from build123d import *

# Parameters (mm, degrees)
F0_R          = 3
F1_DEPTH      = 61
F1_DEPTH_BACK = 4
F0_R_2        = 5
F2_DEPTH      = 55
F5_D          = 2.5
F5_DEPTH      = 8
F5_TIP        = 0.7510757738
F6_D          = 3.5
F6_DEPTH      = 8
F6_TIP        = 1.0515060833


with BuildPart() as f1:
    # F0 (on Top) → F1 (new body, two sides)
    with BuildSketch(Plane.XY) as f1_sk:
        Circle(F0_R)
    extrude(amount=F1_DEPTH)
    extrude(f1_sk.sketch, amount=-F1_DEPTH_BACK)

    # F0 (on Top) → F2 (join)
    with BuildSketch(Plane.XY):
        Circle(F0_R_2)
        Circle(F0_R, mode=Mode.SUBTRACT)
    extrude(amount=F2_DEPTH)

    # F5
    with Locations(Plane(origin=(0, 0, -4), x_dir=(1, 0, 0), z_dir=(0, 0, -1))):
        with Locations((0, 0)):
            Hole(F5_D / 2, depth=F5_DEPTH)
            with Locations((0, 0, -(F5_DEPTH + F5_TIP / 2))):  # 118° drill point
                Cone(0, F5_D / 2, F5_TIP, mode=Mode.SUBTRACT)

    # F6
    with Locations(Plane.XY.offset(61)):
        with Locations((0, 0)):
            Hole(F6_D / 2, depth=F6_DEPTH)
            with Locations((0, 0, -(F6_DEPTH + F6_TIP / 2))):  # 118° drill point
                Cone(0, F6_D / 2, F6_TIP, mode=Mode.SUBTRACT)


solid = f1.part
Part model, mm, in its own coordinate system. A direction names the side the tool comes from. Round coordinates to 2 decimals unless told otherwise and drop trailing zeros. Order: outer loops, then holes, each group sorted by start corner. A loop starts at its lowest first (then second) coordinate and runs counter-clockwise, first axis right, second up. Notation, with made-up numbers: (18.5, 74.5) -> (32.5, 74.5) arc R26 ccw to (32.5, 93.5) -> close; hole circle Ø4 at (-18, -21). An arc over 180 degrees is marked (long way). Put each result on its own line as item: value.
Q1. Pull direction X, two halves, no side cores. Call faces 4 (the face through (-1.617, -0.67, 56.944)), 5 (the face through (-3, 0, 58)), 6 (the face through (-0.1, -3.3, 0)): pulls with the +X half, pulls with the -X half, needs draft (parallel to the pull), parting line crosses it, or undercut.
From the geometry:
face 4: undercut
face 5: parting line crosses it
face 6: needs draft
Q2. Band-saw the part on A-A (z = 26.5). Give the cut face in (x, y).
From the geometry:
outline: circle Ø10 at (0, 0)
Q3. Band-saw the part on B-B (x = 4.25). Give the cut face in (y, z).
From the geometry:
outline: (-2.63, 0) -> (2.63, 0) -> (2.63, 55) -> (-2.63, 55) -> close
Q4. Tool access for faces 1 (the face through (1, -1, -4)), 2 (the face through (0.27, 1.22, 0.06)), 3 (the face through (-0.1, -3.3, 55)): list every direction of +Z, -Z, +X, -X, +Y, -Y with a clear straight run to the whole face (end or side of a thin tool).
From the geometry:
face 1: -Z, +X, -X, +Y, -Y
face 2: -Z
face 3: +Z
Q5. Pin check, flat tips, straight feed: pin 1 Ø2 at (x, y) = (0, 0) entering from +Z; pin 2 Ø1.5 at (y, z) = (-3, 5) entering from -X. Stop position of each tip, or through.
From the geometry:
pin 1: stops at z = 52.55
pin 2: stops at x = -4.47
Q6. Wall check: line 1 (Y direction, x = 0, z = 59.75); line 2 (Z direction, x = 1.25, y = -4); line 3 (X direction, y = -0.25, z = 23). Give the ranges that are in metal, low to high. Write a range as [from, to].
From the geometry:
line 1: y = [-3, -1.75], [1.75, 3]
line 2: z = [0, 55]
line 3: x = [-4.99, 4.99]
